Verification items for the finished model (mm, model axes). A direction names the side the tool comes from. Coordinates: 2 decimals unless noted, no trailing zeros. Order: outer loops, then holes, each group sorted by start corner. A loop starts at its lowest first (then second) coordinate and runs counter-clockwise, first axis right, second up. Notation, with made-up numbers: M -28,11 L 19,11 A16 ccw 19,42 Z; hole C 14.25,36.25 d6. An arc over 180 degrees is marked long. Return JSON: item names as keys, results as strings. Group by question number.
Q1. Section check A-A, the plane z = -3. Enter the section's corners in (x, y).
Q2. Section check B-B, the plane y = 0.5. Enter the section's corners in (x, z).
Q3. Thickness scan on probe 1 along X at (y, z) = (0.45, -3); probe 2 along Y at (x, z) = (5.75, -12); probe 3 along Z at (x, y) = (3, 3.05). Record the ranges inside material, lowest first.
Q4. Section check C-C, the plane x = 3.25. Enter the section's corners in (y, z).
Q5. Go/stop test with flat-tipped pins: pin 1 Ø3.5 at (x, z) = (3.25, -3) entering from +Y; pin 2 Ø0.8 at (x, y) = (1, 2) entering from -Z; pin 3 Ø1.2 at (x, y) = (0.5, 2) entering from +Z. Record where each tip stops, or that it passes through.
Q6. Mould release check, pull along Z, two halves, no side actions. Record for faces 4 (the face through (1.69, 0.39, -3.35)), 5 (the face through (0, 2, -17)), 6 (the face through (-3.5, 2, -15)): pulls with the +Z half, pulls with the -Z half, needs draft (parallel to the pull), parting line crosses it, or undercut.
Q7. Access from +Z, -Z, +X, -X, +Y, -Y to the whole of each face (thin tool, end or side, straight path). Record for faces 1 (the face through (3.5, 2, -15)), 2 (the face through (0, 2, -13)), 3 (the face through (0, 0, -10)).
Q8. Section check D-D, the plane z = -17.75. Enter the section's corners in (x, y), then the cut area to 3 significant figures.
from build123d import *

# Parameters (mm, degrees)
SKETCH1_W           = 12.5
SKETCH1_H           = 20
SKETCH1_R           = 1.6
BOSS_EXTRUDE1_DEPTH = 0.8
SKETCH2_W           = 7
SKETCH2_H           = 4
BOSS_EXTRUDE2_DEPTH = 2.5


with BuildPart() as part:
    # Sketch1 → Boss-Extrude1 (new body)
    with BuildSketch(Plane(origin=(0, 0, 0), x_dir=(1, 0, 0), z_dir=(0, 1, 0))):
        with Locations((0, 10)):
            Rectangle(SKETCH1_W, SKETCH1_H)
        with Locations(Location((3.25, 3, 0), (0, 0, 270))):
            Circle(SKETCH1_R, mode=Mode.SUBTRACT)
    extrude(amount=BOSS_EXTRUDE1_DEPTH)

    # Sketch2 → Boss-Extrude2 (add)
    with BuildSketch(Plane(origin=(0, 0.8, 0), x_dir=(1, 0, 0), z_dir=(0, 1, 0))):
        with Locations((0, 15)):
            Rectangle(SKETCH2_W, SKETCH2_H)
    extrude(amount=BOSS_EXTRUDE2_DEPTH)


solid = part.part
Numbers:
{
 "1": {"outline": "M -6.25,0 L 1.65,0 L 1.65,0.8 L -6.25,0.8 Z; M 4.85,0 L 6.25,0 L 6.25,0.8 L 4.85,0.8 Z"},
 "2": {"outline": "M -6.25,-20 L 6.25,-20 L 6.25,0 L -6.25,0 Z; hole C 3.25,-3 d3.2"},
 "3": {"probe 1": "x = -6.25 to 1.65, 4.85 to 6.25", "probe 2": "y = 0 to 0.8", "probe 3": "z = -17 to -13"},
 "4": {"outline": "M 0,-20 L 0.8,-20 L 0.8,-17 L 3.3,-17 L 3.3,-13 L 0.8,-13 L 0.8,-4.6 L 0,-4.6 Z; M 0,-1.4 L 0.8,-1.4 L 0.8,0 L 0,0 Z"},
 "5": {"pin 1": "stops at y = 0.8", "pin 2": "stops at z = -17", "pin 3": "stops at z = -13"},
 "6": {"face 4": "undercut", "face 5": "pulls with the -Z half", "face 6": "needs draft"},
 "7": {"face 1": "+Z, -Z, +X, +Y", "face 2": "+Z, +X, -X, +Y", "face 3": "+Z, -Z, +X, -X, -Y"},
 "8": {"outline": "M -6.25,0 L 6.25,0 L 6.25,0.8 L -6.25,0.8 Z", "area": "10.0 mm2"}
}
